Geometry check sheet. Reference: the model listing, model coordinates, mm. A direction names the side the tool comes from. Give positions to 0.01 mm unless a question says otherwise; leave off trailing zeros. Order: outer loops, then holes, each group sorted by start corner. A loop starts at its lowest first (then second) coordinate and runs counter-clockwise, first axis right, second up. Notation, with made-up numbers: M -4.75,40.5 L 3.25,40.5 A33 cw 3.25,72.5 Z; hole C 58,71.25 d3. An arc over 180 degrees is marked long. Answer as CSV lines item,"result".
Autodesk Inventor part; units mm, degrees
ref_plane "YZ Plane" through (0, 0, 0) normal (1, 0, 0) x (0, 1, 0)
ref_plane "XZ Plane" through (0, 0, 0) normal (0, 1, 0) x (-1, 0, 0)
ref_plane "XY Plane" through (0, 0, 0) normal (0, 0, 1) x (1, 0, 0)
sketch "Sketch1" plane through (0, 0, 0) normal (0, 0, 1) x (1, 0, 0)
  line L0 (-2.54, -8.19) -> (2.54, -8.19)
  line L1 (2.54, -8.19) -> (2.54, 8.19)
  line L2 (-2.54, 8.19) -> (-2.54, -8.19)
  line L3 (-2.54, -8.19) -> (2.54, 8.19) construction
  line L4 (2.54, -8.19) -> (-2.54, 8.19) construction
  circle A0 centre (0, 16.6545) radius 2.5 construction
  circle A1 centre (0, 16.6545) radius 5
  arc A2 (6.8029, 15.0051) -> (-6.8044, 15.0114) centre (0, 16.6545) ccw
  line L5 (-2.54, 8.19) -> (-2.54, 10.2591)
  line L6 (2.54, 8.19) -> (2.54, 10.2869)
  line L7 (0, 0) -> (0, 10.7842) construction
  line L8 (-2.54, 10.2591) -> (-3.9944, 10.2511)
  line L9 (2.54, 10.2869) -> (3.9944, 10.2948)
  line L10 (-3.9944, 10.2511) -> (-4.1214, 3.9003)
  line L11 (3.9944, 10.2948) -> (4.1214, 3.9454)
  line L12 (-4.1214, 3.9003) -> (-6.8044, 15.0114)
  line L13 (4.1214, 3.9454) -> (6.8029, 15.0051)
  line L14 (0, 0) -> (0, 22.9511) construction
  point P0 (-3.2672, 10.2551)
  dimension "d2" = 5
  dimension "d3" = 10
  dimension "d4" = 14
  dimension "d8" = 1.5815
  dimension "d9" = 1.5815
  dimension "d10" = 6.35
  dimension "d11" = 6.35
  dimension "d18" = 1.4545
  dimension "d19" = 1.4545
  dimension "d31" = 2.54
  dimension "d32" = 2.54
  dimension "d33" = 0
extrude "Plate1" add sketch "Sketch1" along normal blind 3.175
sketch "Sketch2" plane through (0, 0, 0) normal (0, 0, -1) x (-1, 0, 0)
  circle A0 centre (0, 16.6545) radius 5
  line L0 (-3.9944, 10.2948) -> (-4.1214, 3.9454)
  line L1 (-2.54, 10.2869) -> (-3.9944, 10.2948)
  line L2 (-2.54, -8.19) -> (-2.54, 10.2869)
  line L3 (2.54, -8.19) -> (-2.54, -8.19)
  line L4 (2.54, 10.2591) -> (2.54, -8.19)
  line L5 (3.9944, 10.2511) -> (2.54, 10.2591)
  line L6 (4.1214, 3.9003) -> (3.9944, 10.2511)
  line L7 (6.8044, 15.0114) -> (4.1214, 3.9003)
  arc A1 (6.8044, 15.0114) -> (-6.8029, 15.0051) centre (0, 16.6545) ccw
  line L8 (-4.1214, 3.9454) -> (-6.8029, 15.0051)
  line L9 (-1.5875, -17.19) -> (1.5875, -17.19)
  line L10 (1.5875, -17.19) -> (1.5875, 0.81)
  line L11 (1.5875, 0.81) -> (-1.5875, 0.81)
  line L12 (-1.5875, 0.81) -> (-1.5875, -17.19)
  line L13 (-1.5875, -17.19) -> (1.5875, 0.81) construction
  line L14 (1.5875, -17.19) -> (-1.5875, 0.81) construction
  point P0 (0, 0)
  point P1 (0, -8.19)
  dimension "d14" = 3.175
extrude "Extrusion1" cut sketch "Sketch2" against normal blind 25.4 contours L12 L11 L10 L3 | L3 L10 L9 L12
sketch "Sketch3" plane through (0, 0, 3.175) normal (0, 0, 1) x (1, 0, 0)
  circle A0 centre (-37.757, 0) radius 3
  line L0 (-39.3445, -2.5456) -> (-36.1695, -2.5456)
  line L1 (-36.1695, -2.5456) -> (-36.1695, 2.5456)
  line L2 (-36.1695, 2.5456) -> (-39.3445, 2.5456)
  line L3 (-39.3445, 2.5456) -> (-39.3445, -2.5456)
  line L4 (-39.3445, -2.5456) -> (-36.1695, 2.5456) construction
  line L5 (-36.1695, -2.5456) -> (-39.3445, 2.5456) construction
  circle A1 centre (-37.757, 0) radius 4
  point P0 (0, 0)
  point P1 (-37.757, 3)
  point P2 (-37.757, 4)
  dimension "d35" = 8
  dimension "d28" = 6
  dimension "d29" = 3.175
  dimension "d30" = 5.0911
  dimension "d34" = 0.4545
  dimension "d36" = 1.4545
sketch "Sketch4" plane through (0, 0, 3.175) normal (0, 0, 1) x (1, 0, 0)
  line L0 (-1.5875, -8.19) -> (-1.5875, 0.81)
  line L1 (-1.5875, 0.81) -> (1.5875, 0.81)
  line L2 (1.5875, 0.81) -> (1.5875, -8.19)
  line L3 (2.54, -8.19) -> (1.5875, -8.19)
  line L4 (2.54, 10.2869) -> (2.54, -8.19)
  line L5 (3.9944, 10.2948) -> (2.54, 10.2869)
  line L6 (4.1214, 3.9454) -> (3.9944, 10.2948)
  line L7 (6.8029, 15.0051) -> (4.1214, 3.9454)
  arc A0 (6.8029, 15.0051) -> (-6.8044, 15.0114) centre (0, 16.6545) ccw
  line L8 (-4.1214, 3.9003) -> (-6.8044, 15.0114)
  line L9 (-3.9944, 10.2511) -> (-4.1214, 3.9003)
  line L10 (-2.54, 10.2591) -> (-3.9944, 10.2511)
  line L11 (-2.54, -8.19) -> (-2.54, 10.2591)
  line L12 (-1.5875, -8.19) -> (-2.54, -8.19)
  circle A1 centre (0, 16.6545) radius 5
  line L13 (-2.54, 10.2591) -> (-3.7175, 2.2274)
  line L14 (-3.7175, 2.2274) -> (-9.3024, 3.6769)
  line L15 (-9.3024, 3.6769) -> (-11.1796, 30.918)
  line L16 (-11.1796, 30.918) -> (24.5864, 22.2464)
  line L17 (24.5864, 22.2464) -> (4.4395, 2.4617)
  line L18 (4.4395, 2.4617) -> (3.4851, 4.2508)
  line L19 (3.4851, 4.2508) -> (2.54, 10.2869)
  line L20 (2.54, 10.2869) -> (-2.54, 10.2591)
  point P0 (0, 0)
extrude "Extrusion2" cut sketch "Sketch4" against normal blind 25.4 contours L13 L14 L15 L16 L17 L18 L19 L5 L6 L7 A0 L8 L9 L10 | L10 L9 L8 A0 L7 L6 L5 L20 | A1
chamfer "Chamfer3" distance 2.54 angle 10 1 edges at (2.54, 10.2869, 1.5875) measured on face at (2.54, -2.0311, 1.0583)
chamfer "Chamfer4" distance 2.54 angle 10 1 edges at (-2.54, 10.2591, 1.5875) measured on face at (-2.54, -2.0403, 1.0583)
fillet "Fillet5" radius 0.127 4 edges at (-2.0921, 10.2615, 1.5875) (-2.54, 7.7191, 1.5875) (2.0921, 10.2844, 1.5875) (2.54, 7.7469, 1.5875)
fillet "Fillet6" radius 1.5748 2 edges at (-1.5875, 0.81, 1.5875) (1.5875, 0.81, 1.5875)
sketch "Sketch5" plane through (0, 0, 3.175) normal (0, 0, 1) x (1, 0, 0)
  arc A0 (2.54, 7.7358) -> (2.5381, 7.7578) centre (2.413, 7.7358) ccw
  line L0 (2.1112, 10.1789) -> (2.5381, 7.7578)
  arc A1 (2.1112, 10.1789) -> (1.9854, 10.2839) centre (1.9861, 10.1569) ccw
  line L1 (1.9854, 10.2839) -> (-1.9857, 10.2621)
  arc A2 (-1.9857, 10.2621) -> (-2.1101, 10.1572) centre (-1.985, 10.1351) ccw
  line L2 (-2.5381, 7.73) -> (-2.1101, 10.1572)
  arc A3 (-2.5381, 7.73) -> (-2.54, 7.708) centre (-2.413, 7.708) ccw
  line L3 (-2.54, -8.19) -> (-2.54, 7.708)
  line L4 (-1.5875, -8.19) -> (-2.54, -8.19)
  line L5 (-1.5875, -8.19) -> (-1.5875, -0.7648)
  arc A4 (-0.0127, 0.81) -> (-1.5875, -0.7648) centre (-0.0127, -0.7648) ccw
  line L6 (-0.0127, 0.81) -> (0.0127, 0.81)
  arc A5 (1.5875, -0.7648) -> (0.0127, 0.81) centre (0.0127, -0.7648) ccw
  line L7 (1.5875, -0.7648) -> (1.5875, -8.19)
  line L8 (2.54, -8.19) -> (1.5875, -8.19)
  line L9 (2.54, 7.7358) -> (2.54, -8.19)
  circle A6 centre (-2.54, -8.19) radius 0.0635
  circle A7 centre (-1.5875, -8.19) radius 0.0635
  circle A8 centre (1.5875, -8.19) radius 0.0635
  circle A9 centre (2.54, -8.19) radius 0.0635
  point P0 (0, 0)
  dimension "d48" = 0.127
  dimension "d49" = 0.127
  dimension "d50" = 0.127
  dimension "d51" = 0.127
extrude "Extrusion3" add sketch "Sketch5" against normal up to surface (3.175 mm away) contours A9 L8 L9 | L9 L8 A9 | A8 L7 L8 | L8 L7 A8 | A6 L4 L3 | L3 L4 A6 | A7 L4 L5 | L5 L4 A7
fillet "Fillet7" radius 0.0508 8 edges at (-1.651, -8.19, 1.5875) (-2.4765, -8.19, 1.5875) (-2.54, -8.1265, 1.5875) (-1.5875, -8.1265, 1.5875) (2.54, -8.1265, 1.5875) (1.651, -8.19, 1.5875) (1.5875, -8.1265, 1.5875) (2.4765, -8.19, 1.5875)
equation "\"d18\" = d36"
equation "\"d19\" = d36"
equation "\"d49\" = d48"
equation "\"d50\" = d48"
equation "\"d51\" = d48"
equation "\"BendRadius\" = Thickness"
equation "\"BendReliefWidth\" = Thickness"
equation "\"BendReliefDepth\" = 0.5 * Thickness"
equation "\"CornerReliefSize\" = 4 * Thickness"
equation "\"MinimumRemnant\" = 2 * Thickness"
equation "\"TransitionRadius\" = BendRadius"
equation "\"JacobiRadiusSize\" = BendRadius"
equation "\"GapSize\" = Thickness"
equation "\"d12\" = BendRadius"
properties part number "8mm OD 6mm ID Rod Cross125"
(1) Material ranges on line 1 (X direction, y = -3.5, z = 0.7); line 2 (Y direction, x = 1.95, z = 1.15); line 3 (X direction, y = 3, z = 0.85), recorded low to high.
The answers:
line 1,"x = -2.54 to -1.59, 1.59 to 2.54"
line 2,"y = -8.19 to 10.28"
line 3,"x = -2.54 to 2.54"
(2) Gauge pin test, flat end, axial feed: P1, Ø1, axis at y = -3, z = 2, coming from the -X side. Record the tip position at first contact, or that the pin passes through.
The answers:
P1,"stops at x = -2.54"
(3) Section check C-C on y = 2.75. Enter the section's corners in (x, z) (3 decimals).
The answers:
outline,"M -2.54,0 L 2.54,0 L 2.54,3.175 L -2.54,3.175 Z"
(4) Section check D-D on x = -0.5. Enter the section's corners in (y, z) (3 decimals).
The answers:
outline,"M 0.733,0 L 10.27,0 L 10.27,3.175 L 0.733,3.175 Z"
(5) Tool access check on faces 4 (the face through (-2.54, 0, 2)), 5 (the face through (-1.588, -4, 2)), 6 (the face through (2.32, 8.99, 1.57)). Record the directions out of +Z, -Z, +X, -X, +Y, -Y that give a thin tool (end or side, any length) a straight path to the whole face; none if there is none.
The answers:
face 4,"+Z, -Z, -X, +Y"
face 5,"+Z, -Z"
face 6,"+Z, -Z, +X, +Y"
(6) Draft check along Z on faces 1 (the face through (0, 3, 0)), 2 (the face through (0, 3, 3.175)), 3 (the face through (2.54, 0, 2)). Enter one of: +Z half, -Z half, draft (parallel to the pull), parting line (faces both ways), or undercut.
The answers:
face 1,"-Z half"
face 2,"+Z half"
face 3,"draft"
(7) Section check A-A on y = -6.5. Enter the section's corners in (x, z) (1 decimal).
The answers:
outline,"M -2.5,0 L -1.6,0 L -1.6,3.2 L -2.5,3.2 Z; M 1.6,0 L 2.5,0 L 2.5,3.2 L 1.6,3.2 Z"
